from build123d import *

# Parameters (mm, degrees)
CROQUIS1_R              = 1.75
SALIENTE_EXTRUIR1_DEPTH = 2.5


with BuildPart() as part:
    # Croquis1 → Saliente-Extruir1 (new, symmetric)
    with BuildSketch(Plane.XY):
        with BuildLine():
            Line((0, -4), (-4, -4))
            Line((-4, -4), (-4, -1.5))
            Line((-4, -1.5), (-6.5, -1.5))
            Line((-6.5, -1.5), (-6.5, 1.5))
            Line((-6.5, 1.5), (-4, 1.5))
            Line((-4, 1.5), (-4, 4))
            Line((-4, 4), (0, 4))
            ThreePointArc((0, 4), (4, 0), (0, -4))
        make_face()
        Circle(CROQUIS1_R, mode=Mode.SUBTRACT)
    extrude(amount=SALIENTE_EXTRUIR1_DEPTH, both=True)


solid = part.part
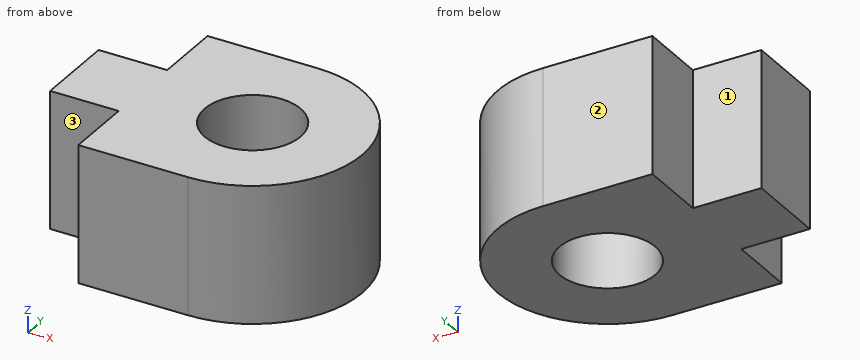
Geometry: final body of the model. Coordinates: model frame, mm. Face numbers are marked on the shaded views. A direction names the side the tool comes from. Coordinates: 2 decimals unless noted, no trailing zeros. Write each loop counter-clockwise with the first axis right and the second up, starting at its lowest first coordinate (ties: lowest second). Pieces come first, ordered by that corner, then holes. Notation, with made-up numbers: (6, -0.75) - (61, -0.75) arc R17 cw to (61, 12.25) - close; hole circle Ø6 at (17.5, 83.5). An arc over 180 degrees is marked (long way). Return JSON: item names as keys, results as strings.
Item 1: Section query C-C (x = -1.25). Output: boundary loops of the cut face in (y, z), and give its area (3 significant figures).
Completed:
{"outline": "(-4, -2.5) - (-1.22, -2.5) - (-1.22, 2.5) - (-4, 2.5) - close; (1.22, -2.5) - (4, -2.5) - (4, 2.5) - (1.22, 2.5) - close", "area": "27.8 mm2"}
Item 2: Reachability of the marked faces 1, 2 and 3 from +Z, -Z, +X, -X, +Y, -Y: full face, straight path, thin tool, end or side. Return the list, or none.
Completed:
{"face 1": "+Z, -Z, -X, +Y", "face 2": "+Z, -Z, +X, -X, +Y", "face 3": "+Z, -Z, -X, -Y"}
Item 3: Pin query (flat end, axial travel): pin 1 Ø2 at (y, z) = (3.5, -0.5) entering from -X; pin 2 Ø0.8 at (x, z) = (-5.5, 0.5) entering from -Y; pin 3 Ø1 at (x, y) = (0, -1) entering from -Z. Return the tip coordinate at first contact, or that it passes through.
Completed:
{"pin 1": "stops at x = -4", "pin 2": "stops at y = -1.5", "pin 3": "passes through"}
Item 4: Section query D-D (x = -5.5). Output: boundary loops of the cut face in (y, z).
Completed:
{"outline": "(-1.5, -2.5) - (1.5, -2.5) - (1.5, 2.5) - (-1.5, 2.5) - close"}
Item 5: Section query A-A (y = 0). Output: boundary loops of the cut face in (x, z), and give its area (3 significant figures).
Completed:
{"outline": "(-6.5, -2.5) - (-1.75, -2.5) - (-1.75, 2.5) - (-6.5, 2.5) - close; (1.75, -2.5) - (4, -2.5) - (4, 2.5) - (1.75, 2.5) - close", "area": "35.0 mm2"}
Item 6: Line query: L1, parallel to X at y = 0.75, z = 0.75; L2, parallel to X at y = -2.75, z = 1.4; L3, parallel to X at y = 0.5, z = 0.2. Output: solid intervals per line, ascending.
Completed:
{"L1": "x = -6.5 to -1.58, 1.58 to 3.93", "L2": "x = -4 to 2.9", "L3": "x = -6.5 to -1.68, 1.68 to 3.97"}
Item 7: Section query B-B (z = 0.7). Output: boundary loops of the cut face in (x, y).
Completed:
{"outline": "(-6.5, -1.5) - (-4, -1.5) - (-4, -4) - (0, -4) arc R4 ccw to (0, 4) - (-4, 4) - (-4, 1.5) - (-6.5, 1.5) - close; hole circle Ø3.5 at (0, 0)"}
